Input: part model. Units: mm. Frame: model coordinates. Face numbers are marked on the shaded views. Round coordinates to 2 decimals unless told otherwise and drop trailing zeros. Loops run counter-clockwise (first coordinate to the right, second up) from the corner with the lowest first, then second, coordinate; pieces in that order, holes last. Notation, with made-up numbers: M 76.25,-10 L 123.25,-10 A24 ccw 123.25,29 Z; hole C 50,44.5 d8. An arc over 180 degrees is marked long. Return JSON: item names as keys, results as strings. Group by question number.
1) Section B-B (x = 0). Output: boundary loops of the cut face in (y, z), plus the area to 3 significant figures.
2) Section A-A (z = 0). Output: boundary loops of the cut face in (x, y), plus the area to 3 significant figures.
3) Material intervals for line 1 (X direction, y = 7.4, z = 0); line 2 (Z direction, x = 0.25, y = 3.75); line 3 (Y direction, x = -0.5, z = 1), sorted ascending. Write a range as from..to.
4) Mould query, pull axis Z, two halves, no side actions, for the marked faces 1, 2, 3 and 4. Classes: +Z half, -Z half, draft (parallel to the pull), parting line (faces both ways), or undercut.
5) Contact query for a flat-ended pin moving along its axis: P1, Ø2.5, axis at x = 0.5, z = 1.5, coming from the +Y side. Output: stop coordinate, or through.
from build123d import *

# Parameters (mm, degrees)
CHAMFER1_SIZE      = 1.75
CHAMFER1_SIZE2     = 0.468911087
SKETCH2_R          = 3
CUT_EXTRUDE1_DEPTH = 16.289865925
CIRPATTERN1_COUNT  = 6
FILLET1_R          = 0.5
CHAMFER2_SIZE      = 0.5


with BuildPart() as part:
    # Sketch1 → Revolve1 (revolve)
    with BuildSketch(Plane(origin=(0, 0, 0), x_dir=(0, 0, -1), z_dir=(1, 0, 0)), mode=Mode.PRIVATE) as revolve1_sk:
        Polygon((0, 0), (-6.7, 0), (-6.7, 12), (-3.7, 12), (-3.7, 4.268512728), (-4.1, 2), (0, 2), align=None)
    revolve(revolve1_sk.sketch.rotate(Axis((0, 0, 0), (0, 1, 0)), 180), axis=Axis((0, 0, 0), (0, 1, 0)))

    # Chamfer1
    chamfer1_edges = [part.edges().sort_by_distance(p)[0] for p in [
        (0, 12, 3.7),
    ]]
    chamfer1_side = [part.faces().sort_by_distance(p)[0] for p in [
        (0, 8.134256364, 3.7),
    ]]
    chamfer(chamfer1_edges, length=CHAMFER1_SIZE, length2=CHAMFER1_SIZE2, reference=chamfer1_side[0])

    # Sketch2 → Cut-Extrude1 (cut, through all)
    with BuildSketch(Plane(origin=(0, 0, 0), x_dir=(1, 0, 0), z_dir=(0, 1, 0))):
        with Locations((0, 8.7)):
            Circle(SKETCH2_R)
    cut_extrude1 = extrude(amount=CUT_EXTRUDE1_DEPTH, mode=Mode.SUBTRACT)

    # CirPattern1: Cut-Extrude1 ×6 about axis
    cirpattern1_axis = Axis((0, 0, 0), (0, 1, 0))
    for i in range(1, CIRPATTERN1_COUNT):
        add(cut_extrude1.rotate(cirpattern1_axis, i * 360 / CIRPATTERN1_COUNT), mode=Mode.SUBTRACT)

    # Fillet1
    fillet1_edges = [part.edges().sort_by_distance(p)[0] for p in [
        (1.941133962, 6, -6.412643678),
        (-1.941133962, 6, -6.412643678),
        (6.524079312, 6, -1.525250516),
        (4.58294535, 6, -4.887393162),
        (4.58294535, 6, 4.887393162),
        (6.524079312, 6, 1.525250516),
        (-1.941133962, 6, 6.412643678),
        (1.941133962, 6, 6.412643678),
        (-6.524079312, 6, 1.525250516),
        (-4.58294535, 6, 4.887393162),
        (-4.58294535, 6, -4.887393162),
        (-6.524079312, 6, -1.525250516),
    ]]
    fillet(fillet1_edges, radius=FILLET1_R)

    # Chamfer2
    chamfer2_edges = [part.edges().sort_by_distance(p)[0] for p in [
        (4.936344802, 0, -2.85),
        (6.7, 0, 0),
        (4.936344802, 0, 2.85),
        (3.35, 0, 5.802370205),
        (0, 0, 5.7),
        (-3.35, 0, 5.802370205),
        (-4.936344802, 0, 2.85),
        (-6.7, 0, 0),
        (-4.936344802, 0, -2.85),
        (-3.35, 0, -5.802370205),
        (0, 0, -5.7),
        (3.35, 0, -5.802370205),
        (-4.515588694, 0, -4.878854752),
        (4.515588694, 0, -4.878854752),
        (1.96741781, 0, -6.350041898),
        (-1.96741781, 0, -6.350041898),
        (-6.483006504, 0, -1.471187146),
        (-6.483006504, 0, 1.471187146),
        (-4.515588694, 0, 4.878854752),
        (-1.96741781, 0, 6.350041898),
        (1.96741781, 0, 6.350041898),
        (4.515588694, 0, 4.878854752),
        (6.483006504, 0, 1.471187146),
        (6.483006504, 0, -1.471187146),
    ]]
    chamfer(chamfer2_edges, length=CHAMFER2_SIZE - 0.0001)  # a hair under: the kernel refuses the full size


solid = part.part
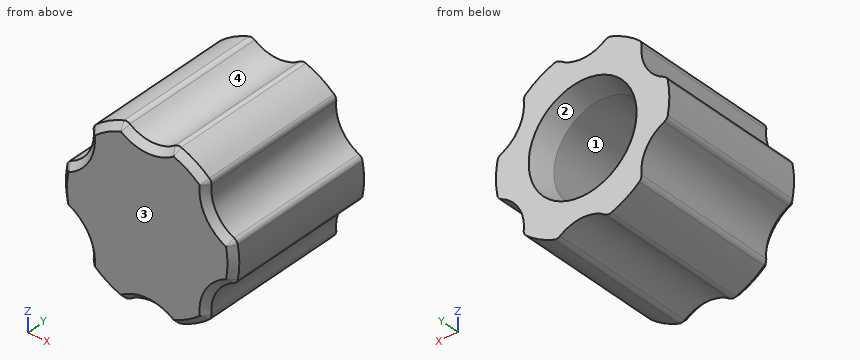
Returned:
{
 "1": {"outline": "M 0,-5.2 L 0.5,-5.7 L 12,-5.7 L 12,-4.17 L 10.25,-3.7 L 4.27,-3.7 L 2,-4.1 L 2,4.1 L 4.27,3.7 L 10.25,3.7 L 12,4.17 L 12,5.7 L 0.5,5.7 L 0,5.2 Z", "area": "60.8 mm^2"},
 "2": {"outline": "M -6.7,0.5 L -6.2,0 L 6.2,0 L 6.7,0.5 L 6.7,12 L 4.17,12 L 3.7,10.25 L 3.7,4.27 L 4.1,2 L -4.1,2 L -3.7,4.27 L -3.7,10.25 L -4.17,12 L -6.7,12 Z", "area": "84.8 mm^2"},
 "3": {"line 1": "x = -6.7..-3.7, 3.7..6.7", "line 2": "z = -5.71..-3.78, 3.78..5.71", "line 3": "y = 0..2"},
 "4": {"face 1": "undercut", "face 2": "undercut", "face 3": "draft", "face 4": "+Z half"},
 "5": {"P1": "stops at y = 2"}
}
